Design review of the part shown in the three views and the two pictorial views. Dimensions are in mm from the part's minimum x, y and z. Round coordinates to 2 decimals unless told otherwise and drop trailing zeros. Loops run counter-clockwise (first coordinate to the right, second up) from the corner with the lowest first, then second, coordinate; pieces in that order, holes last. Notation, with made-up numbers: M 62.25,-34 L 85.25,-34 A21 cw 85.25,0 Z; hole C 78,65.25 d7. An arc over 180 degrees is marked long. Return JSON: item names as keys, results as strings. Group by question number.
Q1. Clearance check with a flat-ended pin moving along its axis: pin 1 Ø1.5 at (x, y) = (25, 75) entering from -Z (1 decimal). State where the tip first meets the part, or that it passes through.
Q2. To check wall thickness, follow line 1 along X through (y, z) = (64.5, 1.75); line 2 along Y through (x, z) = (25, 5.25); line 3 along Y through (x, z) = (22, 3.25). State the ranges of each line that lie inside material, in increasing order.
Q3. Consider section A-A (x = 28.5). State the section outline as (y, z) points.
Q4. Consider section B-B (y = 65). State the section outline as (x, z) points.
Q5. Draft analysis for pull direction X (two halves, no side actions). For the marked faces 1, 2 and 3, state which applies: pulls with the +X half, pulls with the -X half, needs draft (parallel to the pull), parting line crosses it, or undercut.
Q6. Consider section C-C (z = 3.75). State the section outline as (x, y) points, and give its area (3 significant figures).
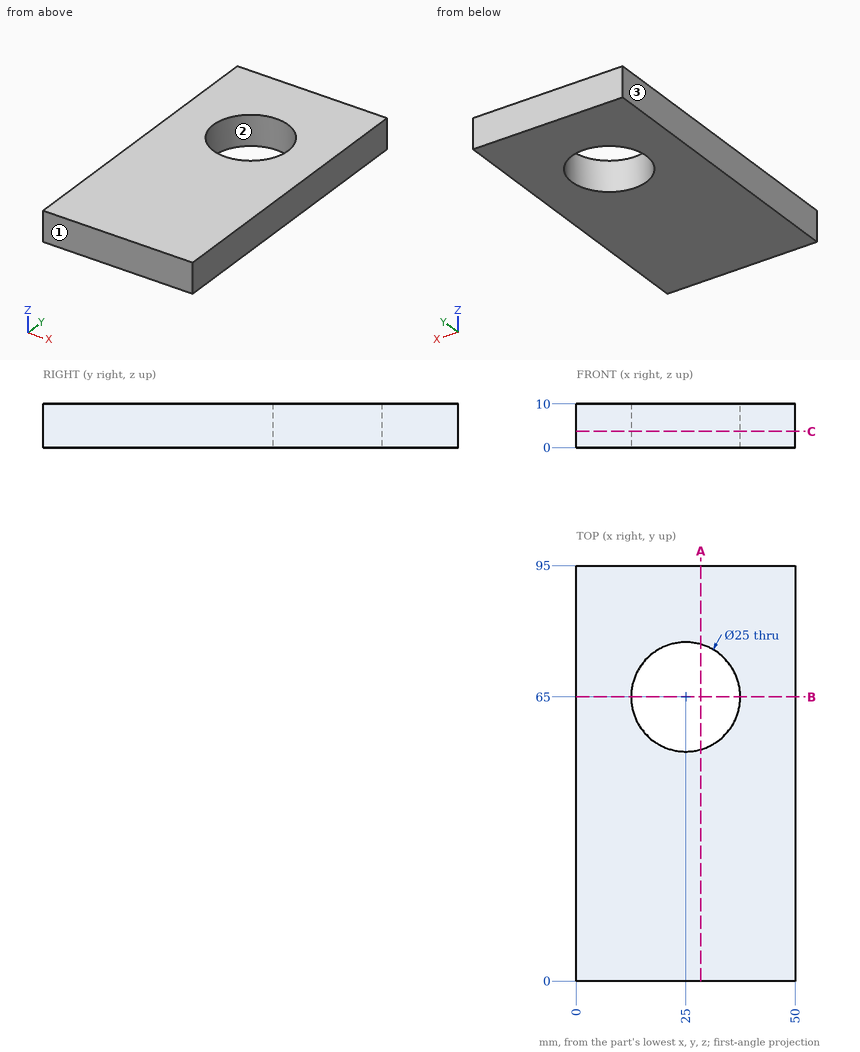
Values:
{
 "1": {"pin 1": "passes through"},
 "2": {"line 1": "x = 0 to 12.51, 37.49 to 50", "line 2": "y = 0 to 52.5, 77.5 to 95", "line 3": "y = 0 to 52.87, 77.13 to 95"},
 "3": {"outline": "M 0,0 L 53,0 L 53,10 L 0,10 Z; M 77,0 L 95,0 L 95,10 L 77,10 Z"},
 "4": {"outline": "M 0,0 L 12.5,0 L 12.5,10 L 0,10 Z; M 37.5,0 L 50,0 L 50,10 L 37.5,10 Z"},
 "5": {"face 1": "needs draft", "face 2": "undercut", "face 3": "pulls with the -X half"},
 "6": {"outline": "M 0,0 L 50,0 L 50,95 L 0,95 Z; hole C 25,65 d25", "area": "4,260 mm2"}
}
